Design review of the part built by this model. Coordinates are the model's own, in mm. A direction names the side the tool comes from. Coordinates: 2 decimals unless noted, no trailing zeros. Loops run counter-clockwise (first coordinate to the right, second up) from the corner with the lowest first, then second, coordinate; pieces in that order, holes last. Notation, with made-up numbers: (38.25, -1) -> (82.25, -1) arc R20 ccw to (82.25, 9) -> close; hole circle Ø9 at (-18, 50.5). An arc over 180 degrees is marked (long way). Use one line per item in the form item = value. Start each with the question number.
1. Wall thickness on line 1 (X direction, y = -8.5, z = 3.45); line 2 (X direction, y = -13, z = 3.85); line 3 (X direction, y = 2.5, z = 4.3): over which ranges is each line inside the solid? List them lowest first. Write a range as from..to.
2. Consider section D-D (x = 0.25). State the section outline as (y, z) points.
3. The part is to be moulded in two halves that separate along Y. For faces 1 (the face through (-5, -0.4, 2.5)), 2 (the face through (-14.327, -5, 2)), 3 (the face through (12, -10.438, 2)), say which applies: released by +Y, released by -Y, zero draft, split by the parting line, or undercut.
4. For pin 1 (5 mm diameter, centred on x = -0.5, y = -4, fed in from +Z); pin 2 (1.5 mm diameter, centred on y = -12.5, z = 3.5, fed in from -X); pin 3 (2.5 mm diameter, centred on y = -14, z = 3, fed in from +X); pin 4 (1.8 mm diameter, centred on x = 5, y = 5.56, fed in from +Z), all flat-tipped, find the tip position at first contact; note any pin that passes through.
5. Consider section A-A (y = -12). State the section outline as (x, z) points, then the cut area to 3 significant figures.
6. Machinability: for faces 4 (the face through (-3, -10.438, 2)), 5 (the face through (-12, -10.438, 2)), 6 (the face through (-2, -7.438, 2)), which of the approach directions +Z, -Z, +X, -X, +Y, -Y give a long, thin tool a straight path to every point of the face, cutting with its end or side? Answer none if there is none.
7. Consider section C-C (y = -1.75). State the section outline as (x, z) points, then the cut area to 3 significant figures.
8. Consider section B-B (z = 1.1). State how many separate pieces and enclosed holes the cut face has, then the cut area to 3 significant figures.
from build123d import *

# Parameters (mm, degrees)
SKETCH1_R           = 1
SKETCH1_W           = 5
SKETCH1_H           = 5
BOSS_EXTRUDE1_DEPTH = 5
FILLET1_R           = 10


with BuildPart() as part:
    # Sketch1 → Boss-Extrude1 (new body)
    # profile 1 of 3: a face of its own
    with BuildSketch(Plane.XY):
        Polygon((-14.326662673, 10.43799709), (-14.326662673, -10.43799709), (-10, -10.43799709), (-5, -10.43799709), (-1.5, -10.43799709), (-1.5, -7.43799709), (-2.6, -7.43799709), (-2.6, -5.13799709), (-1.5, -5.13799709), (-1.5, -0.43799709), (1.5, -0.43799709), (1.5, -5.13799709), (2.6, -5.13799709), (2.6, -7.43799709), (1.5, -7.43799709), (1.5, -10.43799709), (5, -10.43799709), (10, -10.43799709), (14.326662673, -10.43799709), (14.326662673, 10.43799709), align=None)
        with Locations((-5, -3.43799709)):
            Circle(SKETCH1_R, mode=Mode.SUBTRACT)
        with Locations((4, -3.43799709)):
            Circle(SKETCH1_R, mode=Mode.SUBTRACT)
        with Locations((-4, -0.43799709)):
            Circle(SKETCH1_R, mode=Mode.SUBTRACT)
        with Locations((-5, 2.56200291)):
            Circle(SKETCH1_R, mode=Mode.SUBTRACT)
        with Locations((-4, 5.56200291)):
            Circle(SKETCH1_R, mode=Mode.SUBTRACT)
        with Locations((5, -0.43799709)):
            Circle(SKETCH1_R, mode=Mode.SUBTRACT)
        with Locations((4, 2.56200291)):
            Circle(SKETCH1_R, mode=Mode.SUBTRACT)
        with Locations((5, 5.56200291)):
            Circle(SKETCH1_R, mode=Mode.SUBTRACT)
    # profile 2 of 3: a face of its own
    with BuildSketch(Plane.XY):
        with Locations((-7.5, -12.93799709)):
            Rectangle(SKETCH1_W, SKETCH1_H)
    # profile 3 of 3: a face of its own
    with BuildSketch(Plane.XY):
        with Locations((7.5, -12.93799709)):
            Rectangle(SKETCH1_W, SKETCH1_H)
    extrude(amount=BOSS_EXTRUDE1_DEPTH)

    # Fillet1
    fillet1_edges = [part.edges().sort_by_distance(p)[0] for p in [
        (-14.326662673, 10.43799709, 2.5),
        (14.326662673, 10.43799709, 2.5),
    ]]
    fillet(fillet1_edges, radius=FILLET1_R)


solid = part.part
Geometry check:
q1.line_1 = -14.33..-1.5, 1.5..14.33
q1.line_2 = -10..-5, 5..10
q1.line_3 = -14.11..-6, -4..3, 5..14.11
q2.outline = (-0.44, 0) -> (10.44, 0) -> (10.44, 5) -> (-0.44, 5) -> close
q3.face_1 = undercut
q3.face_2 = zero draft
q3.face_3 = released by -Y
q4.pin_1 = 5
q4.pin_2 = -10
q4.pin_3 = 10
q4.pin_4 = through
q5.outline = (-10, 0) -> (-5, 0) -> (-5, 5) -> (-10, 5) -> close; (5, 0) -> (10, 0) -> (10, 5) -> (5, 5) -> close
q5.area = 50.0 mm²
q6.face_4 = +Z, -Z, -Y
q6.face_5 = +Z, -Z, -X, -Y
q6.face_6 = +Z, -Z
q7.outline = (-14.33, 0) -> (-1.5, 0) -> (-1.5, 5) -> (-14.33, 5) -> close; (1.5, 0) -> (14.33, 0) -> (14.33, 5) -> (1.5, 5) -> close
q7.area = 128 mm²
q8.separate_pieces = 1
q8.enclosed_holes = 8
q8.area = 545 mm²
